from build123d import *

# Parameters (mm, degrees)
ESQUISSE1_W             = 258
ESQUISSE1_H             = 148
ESQUISSE1_R             = 1.5
ESQUISSE1_R_2           = 2.5
BOSS_EXTRU_2_DEPTH      = 10
ESQUISSE1_5_W           = 258
ESQUISSE1_5_H           = 148
BOSS_EXTRU_3_DEPTH      = 4
ESQUISSE2_W             = 258
ESQUISSE2_H             = 148
ESQUISSE2_R             = 2.5
BOSS_EXTRU_5_DEPTH      = 40
ENL_V_MAT_EXTRU_1_REACH = 6
ESQUISSE4_W             = 12
ESQUISSE4_H             = 12
ENL_V_MAT_EXTRU_2_REACH = 6
ENL_V_MAT_EXTRU_3_REACH = 6


with BuildPart() as part:
    # Esquisse1 → Boss.-Extru.2 (new body)
    with BuildSketch(Plane.XY):
        Rectangle(ESQUISSE1_W, ESQUISSE1_H)
        with BuildLine():
            Line((-113.5, 67.5), (-113.5, 59.372281323))
            ThreePointArc((-113.5, 59.372281323), (-113.974873734, 58.974873734), (-114.372281323, 58.5))
            Line((-114.372281323, 58.5), (-122.5, 58.5))
            Line((-122.5, 58.5), (-113.5, 67.5))
        make_face(mode=Mode.SUBTRACT)
        with BuildLine():
            Line((-125, 54.5), (-114.372281323, 54.5))
            ThreePointArc((-114.372281323, 54.5), (-113.974873734, 54.025126266), (-113.5, 53.627718677))
            Line((-113.5, 53.627718677), (-113.5, -53.627718677))
            ThreePointArc((-113.5, -53.627718677), (-113.974873734, -54.025126266), (-114.372281323, -54.5))
            Line((-114.372281323, -54.5), (-125, -54.5))
            Line((-125, -54.5), (-125, 54.5))
        make_face(mode=Mode.SUBTRACT)
        with BuildLine():
            Line((-122.5, -58.5), (-114.372281323, -58.5))
            ThreePointArc((-114.372281323, -58.5), (-113.974873734, -58.974873734), (-113.5, -59.372281323))
            Line((-113.5, -59.372281323), (-113.5, -67.5))
            Line((-113.5, -67.5), (-122.5, -58.5))
        make_face(mode=Mode.SUBTRACT)
        with BuildLine():
            Line((-109.5, -70), (-109.5, -59.372281323))
            ThreePointArc((-109.5, -59.372281323), (-109.025126266, -58.974873734), (-108.627718677, -58.5))
            Line((-108.627718677, -58.5), (-2.872281323, -58.5))
            ThreePointArc((-2.872281323, -58.5), (-2.474873734, -58.974873734), (-2, -59.372281323))
            Line((-2, -59.372281323), (-2, -70))
            Line((-2, -70), (-109.5, -70))
        make_face(mode=Mode.SUBTRACT)
        with BuildLine():
            Line((2, -70), (2, -59.372281323))
            ThreePointArc((2, -59.372281323), (2.474873734, -58.974873734), (2.872281323, -58.5))
            Line((2.872281323, -58.5), (108.627718677, -58.5))
            ThreePointArc((108.627718677, -58.5), (109.025126266, -58.974873734), (109.5, -59.372281323))
            Line((109.5, -59.372281323), (109.5, -70))
            Line((109.5, -70), (2, -70))
        make_face(mode=Mode.SUBTRACT)
        with BuildLine():
            Line((113.5, -67.5), (113.5, -59.372281323))
            ThreePointArc((113.5, -59.372281323), (113.974873734, -58.974873734), (114.372281323, -58.5))
            Line((114.372281323, -58.5), (122.5, -58.5))
            Line((122.5, -58.5), (113.5, -67.5))
        make_face(mode=Mode.SUBTRACT)
        with BuildLine():
            Line((125, -54.5), (114.372281323, -54.5))
            ThreePointArc((114.372281323, -54.5), (113.974873734, -54.025126266), (113.5, -53.627718677))
            Line((113.5, -53.627718677), (113.5, 53.627718677))
            ThreePointArc((113.5, 53.627718677), (113.974873734, 54.025126266), (114.372281323, 54.5))
            Line((114.372281323, 54.5), (125, 54.5))
            Line((125, 54.5), (125, -54.5))
        make_face(mode=Mode.SUBTRACT)
        with BuildLine():
            Line((122.5, 58.5), (114.372281323, 58.5))
            ThreePointArc((114.372281323, 58.5), (113.974873734, 58.974873734), (113.5, 59.372281323))
            Line((113.5, 59.372281323), (113.5, 67.5))
            Line((113.5, 67.5), (122.5, 58.5))
        make_face(mode=Mode.SUBTRACT)
        with BuildLine():
            Line((109.5, 70), (109.5, 59.372281323))
            ThreePointArc((109.5, 59.372281323), (109.025126266, 58.974873734), (108.627718677, 58.5))
            Line((108.627718677, 58.5), (2.872281323, 58.5))
            ThreePointArc((2.872281323, 58.5), (2.474873734, 58.974873734), (2, 59.372281323))
            Line((2, 59.372281323), (2, 70))
            Line((2, 70), (109.5, 70))
        make_face(mode=Mode.SUBTRACT)
        with BuildLine():
            Line((-2, 70), (-2, 59.372281323))
            ThreePointArc((-2, 59.372281323), (-2.474873734, 58.974873734), (-2.872281323, 58.5))
            Line((-2.872281323, 58.5), (-108.627718677, 58.5))
            ThreePointArc((-108.627718677, 58.5), (-109.025126266, 58.974873734), (-109.5, 59.372281323))
            Line((-109.5, 59.372281323), (-109.5, 70))
            Line((-109.5, 70), (-2, 70))
        make_face(mode=Mode.SUBTRACT)
        with BuildLine():
            ThreePointArc((2.872281323, -54.5), (2.474873734, -54.025126266), (2, -53.627718677))
            Line((2, -53.627718677), (2, 53.627718677))
            ThreePointArc((2, 53.627718677), (2.474873734, 54.025126266), (2.872281323, 54.5))
            Line((2.872281323, 54.5), (108.627718677, 54.5))
            ThreePointArc((108.627718677, 54.5), (109.025126266, 54.025126266), (109.5, 53.627718677))
            Line((109.5, 53.627718677), (109.5, -53.627718677))
            ThreePointArc((109.5, -53.627718677), (109.025126266, -54.025126266), (108.627718677, -54.5))
            Line((108.627718677, -54.5), (2.872281323, -54.5))
        make_face(mode=Mode.SUBTRACT)
        with BuildLine():
            ThreePointArc((-108.627718677, -54.5), (-109.025126266, -54.025126266), (-109.5, -53.627718677))
            Line((-109.5, -53.627718677), (-109.5, 53.627718677))
            ThreePointArc((-109.5, 53.627718677), (-109.025126266, 54.025126266), (-108.627718677, 54.5))
            Line((-108.627718677, 54.5), (-2.872281323, 54.5))
            ThreePointArc((-2.872281323, 54.5), (-2.474873734, 54.025126266), (-2, 53.627718677))
            Line((-2, 53.627718677), (-2, -53.627718677))
            ThreePointArc((-2, -53.627718677), (-2.474873734, -54.025126266), (-2.872281323, -54.5))
            Line((-2.872281323, -54.5), (-108.627718677, -54.5))
        make_face(mode=Mode.SUBTRACT)
        with Locations((-111.5, 56.5)):
            Circle(ESQUISSE1_R, mode=Mode.SUBTRACT)
        with Locations((0, 56.5)):
            Circle(ESQUISSE1_R, mode=Mode.SUBTRACT)
        with Locations((111.5, 56.5)):
            Circle(ESQUISSE1_R, mode=Mode.SUBTRACT)
        with Locations((-111.5, -56.5)):
            Circle(ESQUISSE1_R, mode=Mode.SUBTRACT)
        with Locations((0, -56.5)):
            Circle(ESQUISSE1_R, mode=Mode.SUBTRACT)
        with Locations((111.5, -56.5)):
            Circle(ESQUISSE1_R, mode=Mode.SUBTRACT)
        with Locations((-121.8320772, -66.8320772)):
            Circle(ESQUISSE1_R_2, mode=Mode.SUBTRACT)
        with Locations((121.8320772, -66.8320772)):
            Circle(ESQUISSE1_R_2, mode=Mode.SUBTRACT)
        with Locations((-121.8320772, 66.8320772)):
            Circle(ESQUISSE1_R_2, mode=Mode.SUBTRACT)
        with Locations((121.8320772, 66.8320772)):
            Circle(ESQUISSE1_R_2, mode=Mode.SUBTRACT)
    extrude(amount=BOSS_EXTRU_2_DEPTH)

    # Esquisse1_5 → Boss.-Extru.3 (add)
    with BuildSketch(Plane.XY):
        Rectangle(ESQUISSE1_5_W, ESQUISSE1_5_H)
    extrude(amount=-BOSS_EXTRU_3_DEPTH)

    # Esquisse2 → Boss.-Extru.5 (add)
    with BuildSketch(Plane.XY.offset(10)):
        Rectangle(ESQUISSE2_W, ESQUISSE2_H)
        with Locations((-121.8320772, 66.8320772)):
            Circle(ESQUISSE2_R, mode=Mode.SUBTRACT)
        with Locations((-121.8320772, -66.8320772)):
            Circle(ESQUISSE2_R, mode=Mode.SUBTRACT)
        with Locations((121.8320772, -66.8320772)):
            Circle(ESQUISSE2_R, mode=Mode.SUBTRACT)
        with Locations((121.8320772, 66.8320772)):
            Circle(ESQUISSE2_R, mode=Mode.SUBTRACT)
        Polygon((-111, 70), (111, 70), (125, 56), (125, -56), (111, -70), (-111, -70), (-125, -56), (-125, 56), align=None, mode=Mode.SUBTRACT)
    extrude(amount=BOSS_EXTRU_5_DEPTH)

    # Esquisse4 → Enl_v. mat.-Extru.1 (cut, up to next)
    with BuildSketch(Plane(origin=(-125, 0, 0), x_dir=(0, 0, -1), z_dir=(1, 0, 0)), mode=Mode.PRIVATE) as enl_v_mat_extru_1_sk1:
        with Locations((-28, 0)):
            Rectangle(ESQUISSE4_W, ESQUISSE4_H)
    enl_v_mat_extru_1_tool1 = extrude(enl_v_mat_extru_1_sk1.sketch, amount=-ENL_V_MAT_EXTRU_1_REACH, mode=Mode.PRIVATE) & part.part
    add(enl_v_mat_extru_1_tool1.solids().sort_by_distance((-125, 0, 28))[0], mode=Mode.SUBTRACT)

    # Esquisse6 → Enl_v. mat.-Extru.2 (cut, up to next)
    with BuildSketch(Plane(origin=(0, -70, 0), x_dir=(1, 0, 0), z_dir=(0, 1, 0)), mode=Mode.PRIVATE) as enl_v_mat_extru_2_sk1:
        with BuildLine():
            Line((10, -40), (10, -50))
            Line((10, -50), (-10, -50))
            Line((-10, -50), (-10, -40))
            ThreePointArc((-10, -40), (0, -30), (10, -40))
        make_face()
    enl_v_mat_extru_2_tool1 = extrude(enl_v_mat_extru_2_sk1.sketch, amount=-ENL_V_MAT_EXTRU_2_REACH, mode=Mode.PRIVATE) & part.part
    add(enl_v_mat_extru_2_tool1.solids().sort_by_distance((0, -70, 40.933499))[0], mode=Mode.SUBTRACT)

    # Esquisse9 → Enl_v. mat.-Extru.3 (cut, up to next)
    with BuildSketch(Plane.XZ.offset(-70), mode=Mode.PRIVATE) as enl_v_mat_extru_3_sk1:
        with BuildLine():
            Line((-10, 40), (-10, 50))
            Line((-10, 50), (10, 50))
            Line((10, 50), (10, 40))
            ThreePointArc((10, 40), (0, 30), (-10, 40))
        make_face()
    enl_v_mat_extru_3_tool1 = extrude(enl_v_mat_extru_3_sk1.sketch, amount=-ENL_V_MAT_EXTRU_3_REACH, mode=Mode.PRIVATE) & part.part
    add(enl_v_mat_extru_3_tool1.solids().sort_by_distance((0, 70, 40.933499))[0], mode=Mode.SUBTRACT)


solid = part.part
CAD build for the part. Positions are in the model's coordinates, mm. A direction names the side the tool comes from. Coordinates: 2 decimals unless noted, no trailing zeros. Write each loop counter-clockwise with the first axis right and the second up, starting at its lowest first coordinate (ties: lowest second). Pieces come first, ordered by that corner, then holes. Notation, with made-up numbers: (64.25, 37.25) - (122.25, 37.25) arc R20 cw to (122.25, 58.25) - close; hole circle Ø1 at (84, 64). An arc over 180 degrees is marked (long way). Use a Markdown table: item, result. Add a question column.
Item 1: Band-saw the part on B-B, the plane z = 45. Give the cut face in (x, y).
Item 2: Band-saw the part on D-D, the plane y = 27. Give the cut face in (x, z).
Item 3: Band-saw the part on A-A, the plane y = -2. Give the cut face in (x, z).
Item 4: Band-saw the part on C-C, the plane x = 16. Give the cut face in (y, z), and give its area (3 significant figures).
Item 5: Flat gauge pins, fed straight in: pin 1 (3 mm diameter, centred on x = -121.83, y = 66.83, fed in from +Z); pin 2 (8 mm diameter, centred on x = -31, y = 51, fed in from +Z). Where does each tip first touch, or does it go through?
Item 6: 3-axis set-ups, long thin cutter, end or side, ignore diameter. For faces 5 (the face through (-56, 54.5, 5)), 6 (the face through (-127, 0, 50)): which of +Z, -Z, +X, -X, +Y, -Y reach the whole face in a straight line?
Item 7: Drill centre lines: L1, parallel to X at y = 8, z = 7; L2, parallel to Y at x = 76.5, z = 5; L3, parallel to X at y = 45, z = 28. Where is each one in solid material? Low to high. Write a range as from..to.
Item 8: Mould opens along X. For faces 1 (the face through (-2, 1, -4)), 2 (the face through (-113.5, 63, 5)), 3 (the face through (-129, -1, 17)), 4 (the face through (-118, 58.5, 5)) say: pulls with the +X half, pulls with the -X half, needs draft (parallel to the pull), parting line crosses it, or undercut.
Numbers:
| question | item | result |
|---|---|---|
| 1 | outline | (-129, -74) - (-10, -74) - (-10, -70) - (-111, -70) - (-125, -56) - (-125, 56) - (-111, 70) - (-10, 70) - (-10, 74) - (-129, 74) - close; (10, -74) - (129, -74) - (129, 74) - (10, 74) - (10, 70) - (111, 70) - (125, 56) - (125, -56) - (111, -70) - (10, -70) - close; hole circle Ø5 at (-121.83, -66.83); hole circle Ø5 at (-121.83, 66.83); hole circle Ø5 at (121.83, -66.83); hole circle Ø5 at (121.83, 66.83) |
| 2 | outline | (-129, -4) - (129, -4) - (129, 50) - (125, 50) - (125, 0) - (113.5, 0) - (113.5, 10) - (109.5, 10) - (109.5, 0) - (2, 0) - (2, 10) - (-2, 10) - (-2, 0) - (-109.5, 0) - (-109.5, 10) - (-113.5, 10) - (-113.5, 0) - (-125, 0) - (-125, 50) - (-129, 50) - close |
| 3 | outline | (-129, -4) - (129, -4) - (129, 50) - (125, 50) - (125, 0) - (113.5, 0) - (113.5, 10) - (109.5, 10) - (109.5, 0) - (2, 0) - (2, 10) - (-2, 10) - (-2, 0) - (-109.5, 0) - (-109.5, 10) - (-113.5, 10) - (-113.5, 0) - (-125, 0) - (-125, 22) - (-129, 22) - close; (-129, 34) - (-125, 34) - (-125, 50) - (-129, 50) - close |
| 4 | outline | (-74, -4) - (74, -4) - (74, 50) - (70, 50) - (70, 0) - (58.5, 0) - (58.5, 10) - (54.5, 10) - (54.5, 0) - (-54.5, 0) - (-54.5, 10) - (-58.5, 10) - (-58.5, 0) - (-70, 0) - (-70, 50) - (-74, 50) - close |
| 4 | area | 1,070 mm2 |
| 5 | pin 1 | z = 0 |
| 5 | pin 2 | z = 10 |
| 6 | face 5 | +Z |
| 6 | face 6 | +Z, +X, -X, +Y, -Y |
| 7 | L1 | -129..-125, -113.5..-109.5, -2..2, 109.5..113.5, 125..129 |
| 7 | L2 | -74..-70, -58.5..-54.5, 54.5..58.5, 70..74 |
| 7 | L3 | -129..-125, 125..129 |
| 8 | face 1 | needs draft |
| 8 | face 2 | undercut |
| 8 | face 3 | pulls with the -X half |
| 8 | face 4 | undercut |
